```python
from build123d import *

# Parameters (mm, degrees)
F0_R     = 11
F1_DEPTH = 1
F2_R     = 4
F3_DEPTH = 4
F4_R     = 0.8
F5_R     = 5.25
F5_R_2   = 4
F6_DEPTH = 0.75
F7_R     = 10.1819626288
F7_R_2   = 8.5
F7_R_3   = 7
F7_R_4   = 5.5
F7_R_5   = 4
F7_R_6   = 2.5
F8_DEPTH = 1


with BuildPart() as f1:
    # F0 (on Top) → F1 (new body)
    with BuildSketch(Plane.XY):
        Circle(F0_R)
    extrude(amount=F1_DEPTH)

    # F2 (on face) → F3 (join)
    with BuildSketch(Plane.XY.offset(1)):
        Circle(F2_R)
    extrude(amount=F3_DEPTH)

    # F4
    f4_edges = [f1.edges().sort_by_distance(p)[0] for p in [
        (-11, 0, 0),
        (-4, 0, 5),
    ]]
    fillet(f4_edges, radius=F4_R)

    # F5 (on face) → F6 (join)
    with BuildSketch(Plane.XY.offset(1)):
        Circle(F5_R)
        Circle(F5_R_2, mode=Mode.SUBTRACT)
        Circle(F5_R_2)
    extrude(amount=F6_DEPTH)

    # F7 (on face) → F8 (join)
    with BuildSketch(Plane(origin=(0, 0, 0), x_dir=(1, 0, 0), z_dir=(0, 0, -1))):
        Circle(F7_R)
        Circle(F7_R_2, mode=Mode.SUBTRACT)
        Circle(F7_R_3)
        Circle(F7_R_4, mode=Mode.SUBTRACT)
        Circle(F7_R_5)
        Circle(F7_R_6, mode=Mode.SUBTRACT)
    extrude(amount=F8_DEPTH)


solid = f1.part
```
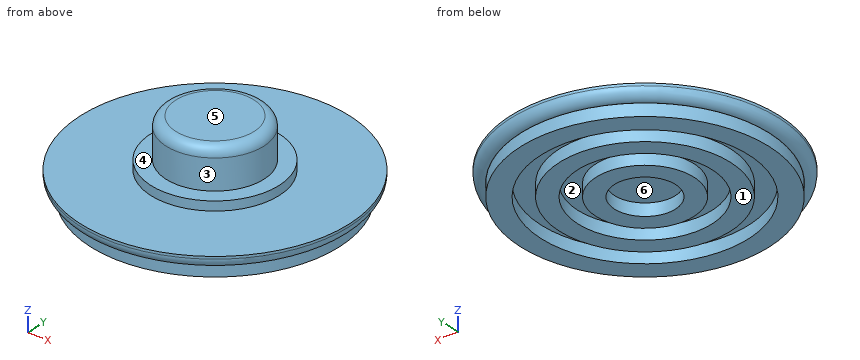
CAD build for the part. Positions are in the model's coordinates, mm. Face numbers are marked on the shaded views. A direction names the side the tool comes from. Round coordinates to 2 decimals unless told otherwise and drop trailing zeros. Use a Markdown table: item, result. Add a question column.
(1) Which spindle directions (+Z, -Z, +X, -X, +Y, -Y) get a long thin tool onto all of the face, cutting with end or side? Do the marked faces 4, 5 and 6. Say none if no direction does.
(2) Drill centre lines: line 1 (Y direction, x = 0, z = -0.6); line 2 (Y direction, x = -2, z = -0.05). Where is each one in solid material? Low to high.
(3) Pull direction Y, two halves, no side cores. Call the marked faces 1, 2 and 3: +Y half, -Y half, draft (parallel to the pull), parting line (faces both ways), or undercut.
(4) Flat gauge pins, fed straight in: pin 1 (1.5 mm diameter, centred on x = 5, z = 2, fed in from +Y); pin 2 (4.5 mm diameter, centred on x = 0, y = 0, fed in from -Z); pin 3 (3 mm diameter, centred on y = -4, z = 1.5, fed in from -X). Where does each tip first touch, or does it go through?
Geometry says:
| question | item | result |
|---|---|---|
| 1 | face 4 | +Z |
| 1 | face 5 | +Z, +X, -X, +Y, -Y |
| 1 | face 6 | -Z |
| 2 | line 1 | y = -10.18 to -8.5, -7 to -5.5, -4 to -2.5, 2.5 to 4, 5.5 to 7, 8.5 to 10.18 |
| 2 | line 2 | y = -9.98 to -8.26, -6.71 to -5.12, -3.46 to -1.5, 1.5 to 3.46, 5.12 to 6.71, 8.26 to 9.98 |
| 3 | face 1 | draft |
| 3 | face 2 | undercut |
| 3 | face 3 | parting line |
| 4 | pin 1 | stops at y = 3.02 |
| 4 | pin 2 | stops at z = 0 |
| 4 | pin 3 | stops at x = -10.69 |
